Check sheet for the modelled part. Datum: model origin and axes. Units: mm. A direction names the side the tool comes from. Round coordinates to 2 decimals unless told otherwise and drop trailing zeros. Order: outer loops, then holes, each group sorted by start corner. A loop starts at its lowest first (then second) coordinate and runs counter-clockwise, first axis right, second up.
(1) Tool access check on faces 4 (the flat face through (-3, -4, 40)), 5 (the flat face through (2, -6, 0)). Record the directions out of +Z, -Z, +X, -X, +Y, -Y that give a thin tool (end or side, any length) a straight path to the whole face; none if there is none.
(2) Mould release check, pull along X, two halves, no side actions. Record for faces 1 (the flat face through (4, 1, -5)), 2 (the cylindrical face through (-6, 0, 20)), 3 (the cylindrical face through (-3.796, -0.167, -2.535)): released by +X, released by -X, zero draft, split by the parting line, or undercut.
(3) Depth check by flat-ended pin: pin 1 (2 mm diameter, centred on y = 1.5, z = 22.5, fed in from +X); pin 2 (8 mm diameter, centred on y = -3, z = 14.5, fed in from -X); pin 3 (8.5 mm diameter, centred on x = 0, y = 0, fed in from -Z); pin 4 (2 mm diameter, centred on x = -3.5, z = 10.5, fed in from +Y). Enter the tip coordinate at first touch or a pass-through.
(4) Thickness scan on probe 1 along Y at (x, z) = (0, 27); probe 2 along X at (y, z) = (0, -3.8); probe 3 along X at (y, z) = (0, -2.6). Record the ranges inside material, lowest first.
(5) Sectioned sample at A-A, the plane x = 0. Enter the section's corners in (y, z).
(6) Sectioned sample at B-B, the plane z = 26. Enter the section's corners in (x, y), and give its area (3 significant figures).
(7) Sectioned sample at C-C, the plane z = -1.5. Enter the section's corners in (x, y).
```python
from build123d import *

# Parameters (mm, degrees)
F0_R     = 6
F0_R_2   = 4.8
F1_DEPTH = 40
F2_R     = 9
F3_DEPTH = 5
F3_TAPER = 35
F4_SIZE  = 1
F5_SIZE  = 0.3
F6_R     = 3.8
F7_DEPTH = 100


with BuildPart() as f1:
    # F0 (on Top) → F1 (new body)
    with BuildSketch(Plane.XY):
        Circle(F0_R)
        Circle(F0_R_2, mode=Mode.SUBTRACT)
    extrude(amount=F1_DEPTH)

    # F2 (on Top) → F3 (join)
    with BuildSketch(Plane.XY):
        Circle(F2_R)
    extrude(amount=-F3_DEPTH, taper=F3_TAPER)

    # F4
    f4_edges = [f1.edges().sort_by_distance(p)[0] for p in [
        (-4.8, 0, 0),
    ]]
    chamfer(f4_edges, length=F4_SIZE)

    # F5
    f5_edges = [f1.edges().sort_by_distance(p)[0] for p in [
        (-6, 0, 40),
    ]]
    chamfer(f5_edges, length=F5_SIZE)

    # F6 (on face) → F7 (cut)
    with BuildSketch(Plane(origin=(0, 0, -5), x_dir=(1, 0, 0), z_dir=(0, 0, -1))):
        Circle(F6_R)
    extrude(amount=-F7_DEPTH, mode=Mode.SUBTRACT)


solid = f1.part
```
Derived:
1. face 4: +Z, +X, -X, +Y, -Y
1. face 5: +Z
2. face 1: zero draft
2. face 2: split by the parting line
2. face 3: undercut
3. pin 1: stops at x = 5.98
3. pin 2: stops at x = -6
3. pin 3: stops at z = -5
3. pin 4: stops at y = 5.45
4. probe 1: y = -6 to -4.8, 4.8 to 6
4. probe 2: x = -6.34 to -3.8, 3.8 to 6.34
4. probe 3: x = -7.18 to -3.8, 3.8 to 7.18
5. outline: (-9, 0) - (-5.5, -5) - (-3.8, -5) - (-3.8, 0) - (-4.8, 1) - (-4.8, 40) - (-5.7, 40) - (-6, 39.7) - (-6, 0) - close; (3.8, -5) - (5.5, -5) - (9, 0) - (6, 0) - (6, 39.7) - (5.7, 40) - (4.8, 40) - (4.8, 1) - (3.8, 0) - close
6. outline: circle Ø12 at (0, 0); hole circle Ø9.6 at (0, 0)
6. area: 40.7 mm2
7. outline: circle Ø15.9 at (0, 0); hole circle Ø7.6 at (0, 0)
